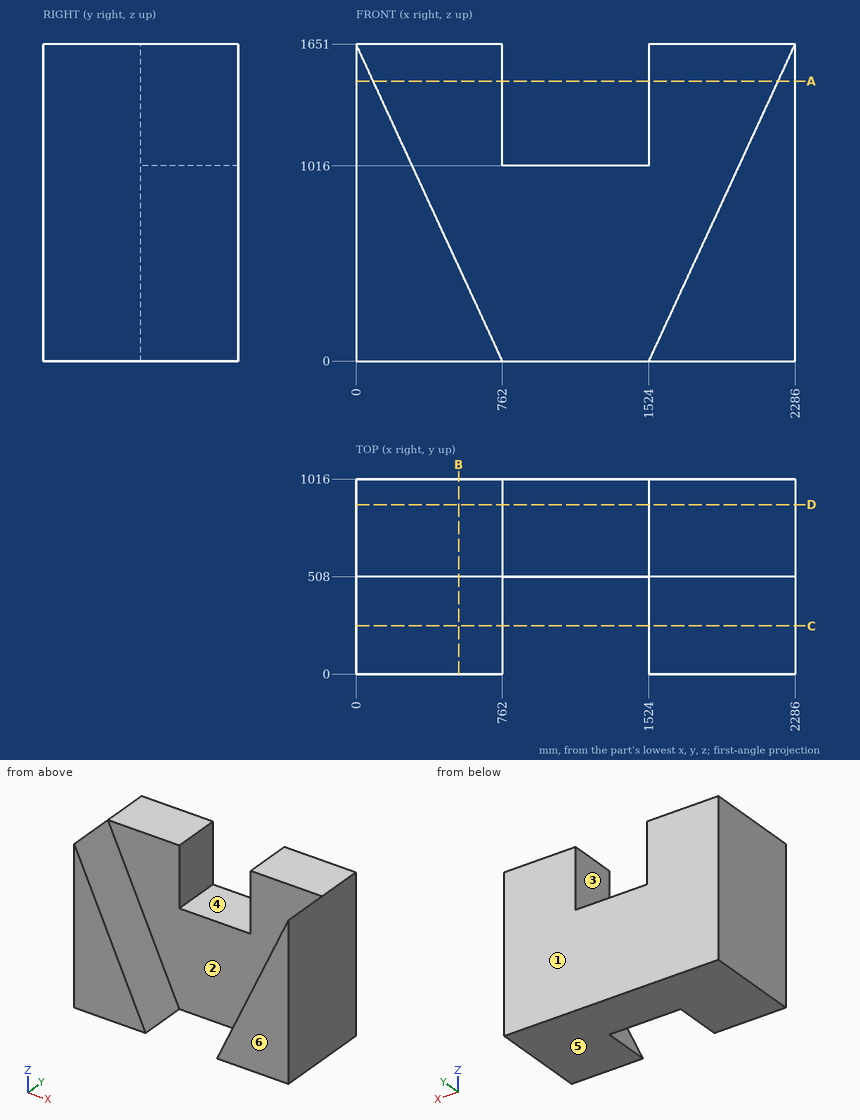
Check sheet for the drawn part. Datum: minimum x, y, z corner. Units: mm. A direction names the side the tool comes from. Coordinates: 2 decimals unless noted, no trailing zeros. Order: outer loops, then holes, each group sorted by start corner. A loop starts at its lowest first (then second) coordinate and runs counter-clockwise, first axis right, second up. Notation, with made-up numbers: (-31, 0) -> (-20, 0) arc R17 cw to (-20, 32) -> close; hole circle Ø9 at (-13.5, 12). An arc over 180 degrees is marked (long way). Use a Markdown table: item, result. Add a question column.
1. Mould release check, pull along Z, two halves, no side actions. Record for the marked faces 4, 5 and 6: pulls with the +Z half, pulls with the -Z half, needs draft (parallel to the pull), parting line crosses it, or undercut.
2. Cross-section at D-D (y = 883). Enter the section's corners in (x, z).
3. Set-up check for the marked faces 1, 2 and 3: record each of +Z, -Z, +X, -X, +Y, -Y from which the full face is reachable in a straight line by a thin tool's end or side.
4. Cross-section at A-A (z = 1457). Enter the section's corners in (x, y), and give its area (3 significant figures).
5. Material ranges on L1, parallel to X at y = 663, z = 1185.5; L2, parallel to Y at x = 523.5, z = 542; L3, parallel to X at y = 227.5, z = 957.5, recorded low to high.
6. Cross-section at B-B (x = 534). Enter the section's corners in (y, z).
7. Cross-section at C-C (y = 251). Enter the section's corners in (x, z), and give its area (3 significant figures).
Filled sheet:
| question | item | result |
|---|---|---|
| 1 | face 4 | pulls with the +Z half |
| 1 | face 5 | pulls with the -Z half |
| 1 | face 6 | needs draft |
| 2 | outline | (0, 0) -> (2286, 0) -> (2286, 1651) -> (1524, 1651) -> (1524, 1016) -> (762, 1016) -> (762, 1651) -> (0, 1651) -> close |
| 3 | face 1 | +Z, -Z, +X, -X, +Y |
| 3 | face 2 | +Z, -Y |
| 3 | face 3 | +Z, +Y, -Y |
| 4 | outline | (0, 0) -> (89.54, 0) -> (89.54, 508) -> (762, 508) -> (762, 1016) -> (0, 1016) -> close; (1524, 508) -> (2196.46, 508) -> (2196.46, 0) -> (2286, 0) -> (2286, 1016) -> (1524, 1016) -> close |
| 4 | area | 865,000 mm2 |
| 5 | L1 | 0 to 762, 1524 to 2286 |
| 5 | L2 | 508 to 1016 |
| 5 | L3 | 0 to 320.08, 1965.92 to 2286 |
| 6 | outline | (0, 0) -> (1016, 0) -> (1016, 1651) -> (508, 1651) -> (508, 494) -> (0, 494) -> close |
| 7 | outline | (0, 0) -> (762, 0) -> (0, 1651) -> close; (1524, 0) -> (2286, 0) -> (2286, 1651) -> close |
| 7 | area | 1,260,000 mm2 |
